Here's how the part is built. I have some questions about the finished solid (model axes, mm). Give positions to 0.01 mm unless a question says otherwise; leave off trailing zeros. Write each loop counter-clockwise with the first axis right and the second up, starting at its lowest first coordinate (ties: lowest second). Pieces come first, ordered by that corner, then holes. Notation, with made-up numbers: (63, -20) - (104, -20) arc R25 ccw to (104, 17) - close; hole circle Ø9 at (89.5, 81). An arc over 180 degrees is marked (long way). Use one line per item in the form item = value. Start each with the question number.
from build123d import *

# Parameters (mm, degrees)
PCB_BASE_DEPTH       = 1.6
SKETCH2_R            = 1.5
MOUNTING_HOLES_DEPTH = 1.6


with BuildPart() as part:
    # Sketch1 → PCB Base (new body)
    with BuildSketch(Plane(origin=(0, 0, 0), x_dir=(1, 0, 0), z_dir=(0, 1, 0))):
        with BuildLine():
            Line((-33.5, -17.5), (33.5, -17.5))
            ThreePointArc((33.5, -17.5), (34.560660172, -17.060660172), (35, -16))
            Line((35, -16), (35, 16))
            ThreePointArc((35, 16), (34.560660172, 17.060660172), (33.5, 17.5))
            Line((33.5, 17.5), (-33.5, 17.5))
            ThreePointArc((-33.5, 17.5), (-34.560660172, 17.060660172), (-35, 16))
            Line((-35, 16), (-35, -16))
            ThreePointArc((-35, -16), (-34.560660172, -17.060660172), (-33.5, -17.5))
        make_face()
    extrude(amount=PCB_BASE_DEPTH)

    # Sketch2 → Mounting Holes (cut)
    with BuildSketch(Plane(origin=(0, 1.6, 0), x_dir=(1, 0, 0), z_dir=(0, 1, 0))):
        with Locations(Location((-32, 14.5, 0), (0, 0, 270))):
            Circle(SKETCH2_R)
        with Locations(Location((32, 14.5, 0), (0, 0, 90))):
            Circle(SKETCH2_R)
        with Locations(Location((32, -14.5, 0), (0, 0, 270))):
            Circle(SKETCH2_R)
        with Locations(Location((-32, -14.5, 0), (0, 0, 90))):
            Circle(SKETCH2_R)
    extrude(amount=-MOUNTING_HOLES_DEPTH, mode=Mode.SUBTRACT)


solid = part.part
1. We'd pull the mould along X, two halves only. Please class faces 1 (the face through (0, 1, 17.5)), 2 (the face through (31.1, 0.8, 13.3)), 3 (the face through (-34.55, 0.79, -17.07)): pulls with the +X half, pulls with the -X half, needs draft (parallel to the pull), parting line crosses it, or undercut.
2. I want a section at A-A, the plane z = -14.5. List the corners of the cut face in (x, y) for me, then the cut area to 3 significant figures.
3. I want a section at B-B, the plane x = 32. List the corners of the cut face in (y, z) for me, then the cut area to 3 significant figures.
4. Please list where these lines run through material, in increasing order: line 1 (X direction, y = 1, z = -14.5); line 2 (X direction, y = 1.35, z = -14).
Result sheet:
q1.face_1 = needs draft
q1.face_2 = undercut
q1.face_3 = pulls with the -X half
q2.outline = (-35, 0) - (-33.5, 0) - (-33.5, 1.6) - (-35, 1.6) - close; (-30.5, 0) - (30.5, 0) - (30.5, 1.6) - (-30.5, 1.6) - close; (33.5, 0) - (35, 0) - (35, 1.6) - (33.5, 1.6) - close
q2.area = 102 mm2
q3.outline = (0, -17.5) - (1.6, -17.5) - (1.6, -16) - (0, -16) - close; (0, -13) - (1.6, -13) - (1.6, 13) - (0, 13) - close; (0, 16) - (1.6, 16) - (1.6, 17.5) - (0, 17.5) - close
q3.area = 46.4 mm2
q4.line_1 = -35 to -33.5, -30.5 to 30.5, 33.5 to 35
q4.line_2 = -35 to -33.41, -30.59 to 30.59, 33.41 to 35
